Geometry check sheet. Reference: the model listing, model coordinates, mm. A direction names the side the tool comes from. Coordinates: 2 decimals unless noted, no trailing zeros. Loops run counter-clockwise (first coordinate to the right, second up) from the corner with the lowest first, then second, coordinate; pieces in that order, holes last. Notation, with made-up numbers: (40.5, -10.75) -> (63.5, -10.75) arc R13 cw to (63.5, 7.25) -> close; hole circle Ø6 at (81, -34). An arc over 180 degrees is marked (long way). Answer as a JSON object with one key per item and string values.
from build123d import *

# Parameters (mm, degrees)
SKETCH1_R           = 12.5
BOSS_EXTRUDE1_DEPTH = 6


with BuildPart() as part:
    # Sketch1 → Boss-Extrude1 (new body)
    with BuildSketch(Plane(origin=(0, 0, 0), x_dir=(1, 0, 0), z_dir=(0, 1, 0))):
        Polygon((-33.710320086, 36.107507173), (-33.710320086, -43.892492827), (-21.830156213, -43.892492827), (-21.830156213, -49.832574764), (-6.979951371, -49.832574764), (-6.979951371, -43.892492827), (12.820321751, -43.892492827), (12.820321751, -49.832574764), (27.670526593, -49.832574764), (27.670526593, -43.892492827), (30.000473961, -43.892492827), (30.000473961, 36.107507173), (27.670526593, 36.107507173), (27.670526593, 42.047589109), (12.820321751, 42.047589109), (12.820321751, 36.107507173), (-6.979951371, 36.107507173), (-6.979951371, 42.047589109), (-21.830156213, 42.047589109), (-21.830156213, 36.107507173), align=None)
        with Locations(Location((0, -3.892492827, 0), (0, 0, 270))):
            Circle(SKETCH1_R, mode=Mode.SUBTRACT)
        with BuildLine():
            Line((-25.103576844, -25.460535765), (-18.032509032, -18.389467953))
            ThreePointArc((-18.032509032, -18.389467953), (-14.496975126, -18.389467953), (-14.496975126, -21.925001859))
            Line((-14.496975126, -21.925001859), (-21.568042938, -28.996069671))
            ThreePointArc((-21.568042938, -28.996069671), (-25.103576844, -28.996069671), (-25.103576844, -25.460535765))
        make_face(mode=Mode.SUBTRACT)
        with BuildLine():
            Line((-21.568042938, 21.211084017), (-14.496975126, 14.140016205))
            ThreePointArc((-14.496975126, 14.140016205), (-14.496975126, 10.604482299), (-18.032509032, 10.604482299))
            Line((-18.032509032, 10.604482299), (-25.103576844, 17.675550111))
            ThreePointArc((-25.103576844, 17.675550111), (-25.103576844, 21.211084017), (-21.568042938, 21.211084017))
        make_face(mode=Mode.SUBTRACT)
        with BuildLine():
            Line((25.103576844, 17.675550111), (18.032509032, 10.604482299))
            ThreePointArc((18.032509032, 10.604482299), (14.496975126, 10.604482299), (14.496975126, 14.140016205))
            Line((14.496975126, 14.140016205), (21.568042938, 21.211084017))
            ThreePointArc((21.568042938, 21.211084017), (25.103576844, 21.211084017), (25.103576844, 17.675550111))
        make_face(mode=Mode.SUBTRACT)
        with BuildLine():
            Line((21.568042938, -28.996069671), (14.496975126, -21.925001859))
            ThreePointArc((14.496975126, -21.925001859), (14.496975126, -18.389467953), (18.032509032, -18.389467953))
            Line((18.032509032, -18.389467953), (25.103576844, -25.460535765))
            ThreePointArc((25.103576844, -25.460535765), (25.103576844, -28.996069671), (21.568042938, -28.996069671))
        make_face(mode=Mode.SUBTRACT)
    extrude(amount=BOSS_EXTRUDE1_DEPTH)


solid = part.part
1. Section check D-D, the plane x = 17. Record the boundary of the cut face in (y, z).
Evaluation:
{"outline": "(0, -42.05) -> (6, -42.05) -> (6, -16.64) -> (0, -16.64) -> close; (0, -9.98) -> (6, -9.98) -> (6, 17.77) -> (0, 17.77) -> close; (0, 24.43) -> (6, 24.43) -> (6, 49.83) -> (0, 49.83) -> close"}
2. Thickness scan on probe 1 along X at (y, z) = (0.5, -14.5); probe 2 along X at (y, z) = (4.2, -18); probe 3 along Z at (x, y) = (-26, 2.3). Record the ranges inside material, lowest first. Write a range as from..to.
Evaluation:
{"probe 1": "x = -33.71..-21.93, -14.86..14.86, 21.93..30", "probe 2": "x = -33.71..-25.38, -18.36..18.36, 25.38..30", "probe 3": "z = -36.11..43.89"}
3. Section check C-C, the plane y = 2.8. State how many separate pieces and enclosed holes the cut face has, then the cut area to 3 significant figures.
Evaluation:
{"separate pieces": "1", "enclosed holes": "5", "area": "4,680 mm^2"}
4. Section check A-A, the plane x = 0. Record the boundary of the cut face in (y, z), then the cut area to 3 significant figures.
Evaluation:
{"outline": "(0, -36.11) -> (6, -36.11) -> (6, -8.61) -> (0, -8.61) -> close; (0, 16.39) -> (6, 16.39) -> (6, 43.89) -> (0, 43.89) -> close", "area": "330 mm^2"}
5. Tool access check on faces 4 (the face through (-28, 3, 43.892)), 5 (the face through (-28, 3, -36.108)), 6 (the face through (12.82, 3, 47)). Record the directions out of +Z, -Z, +X, -X, +Y, -Y that give a thin tool (end or side, any length) a straight path to the whole face; none if there is none.
Evaluation:
{"face 4": "+Z, -X, +Y, -Y", "face 5": "-Z, -X, +Y, -Y", "face 6": "+Z, +Y, -Y"}
6. Section check B-B, the plane z = 1.5. Record the boundary of the cut face in (x, y).
Evaluation:
{"outline": "(-33.71, 0) -> (-12.27, 0) -> (-12.27, 6) -> (-33.71, 6) -> close; (12.27, 0) -> (30, 0) -> (30, 6) -> (12.27, 6) -> close"}
7. Mould release check, pull along Z, two halves, no side actions. Record for faces 1 (the face through (-21.618, 2.958, 21.974)), 2 (the face through (-14, 3, -42.048)), 3 (the face through (20, 3, 49.833)): released by +Z, released by -Z, zero draft, split by the parting line, or undercut.
Evaluation:
{"face 1": "undercut", "face 2": "released by -Z", "face 3": "released by +Z"}
8. Depth check by flat-ended pin: P1, Ø1.8, axis at y = 4.5, z = 48, coming from the -X side; P2, Ø0.7, axis at x = 28.5, y = 2, coming from the +Z side; P3, Ø1.2, axis at x = 29, y = 2, coming from the -Z side; P4, Ø20, axis at x = 0, z = 3.89, coming from the +Y side. Enter the tip coordinate at first touch or a pass-through.
Evaluation:
{"P1": "stops at x = -21.83", "P2": "stops at z = 43.89", "P3": "stops at z = -36.11", "P4": "passes through"}
